from build123d import *

# Parameters (mm, degrees)
ESQUISSE2_R             = 1.2
ENL_V_MAT_EXTRU_1_DEPTH = 16


with BuildPart() as part:
    # Esquisse1 → Révolution1 (revolve)
    with BuildSketch(Plane.XY, mode=Mode.PRIVATE) as r_volution1_sk:
        Polygon((4, 0), (4, -5), (10, -5), (10, -1), (7.75, -1), (7.75, 0), align=None)
    revolve(r_volution1_sk.sketch.rotate(Axis((0, 0, 0), (0, -1, 0)), 180), axis=Axis((0, 0, 0), (0, -1, 0)))

    # Esquisse2 → Enlèv. mat.-Extru.1 (cut, through all)
    with BuildSketch(Plane(origin=(0, 0, 0), x_dir=(1, 0, 0), z_dir=(0, 1, 0))):
        with Locations(Location((6, 0, 0), (0, 0, 180))):
            Circle(ESQUISSE2_R)
        with Locations(Location((-6, 0, 0), (0, 0, 180))):
            Circle(ESQUISSE2_R)
    extrude(amount=-ENL_V_MAT_EXTRU_1_DEPTH, mode=Mode.SUBTRACT)


solid = part.part
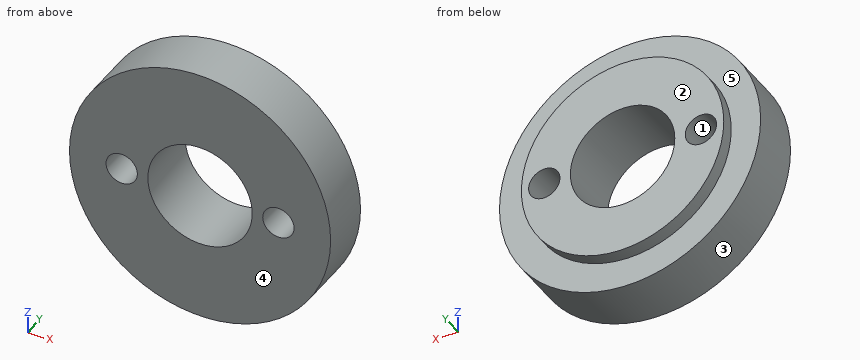
Verification items for the finished model (mm, model axes). Face numbers are marked on the shaded views. A direction names the side the tool comes from. Round coordinates to 2 decimals unless told otherwise and drop trailing zeros. Loops run counter-clockwise (first coordinate to the right, second up) from the corner with the lowest first, then second, coordinate; pieces in that order, holes last. Notation, with made-up numbers: (33, 46) - (68, 46) arc R9 ccw to (68, 61) - close; hole circle Ø6 at (-24, -19.75). An arc over 180 degrees is marked (long way). Use a Markdown table: item, result. Add a question column.
1. Thickness scan on probe 1 along X at (y, z) = (-3.1, 1); probe 2 along Z at (x, y) = (0, -2.75); probe 3 along Y at (x, z) = (-8.25, 3.25). Record the ranges inside material, lowest first. Write a range as [from, to].
2. Section check D-D, the plane y = -2. Record the boundary of the cut face in (x, z).
3. Section check C-C, the plane z = -2. Record the boundary of the cut face in (x, y), plus the area to 3 significant figures.
4. Access from +Z, -Z, +X, -X, +Y, -Y to the whole of each face (thin tool, end or side, straight path). Record for the marked faces 4 and 5.
5. Section check B-B, the plane z = 0. Record the boundary of the cut face in (x, y), plus the area to 3 significant figures.
6. Release check for a two-part mould opening along Z. For the marked faces 1, 2 and 3 record: released by +Z, released by -Z, zero draft, split by the parting line, or undercut.
7. Section check A-A, the plane x = 0. Record the boundary of the cut face in (y, z), plus the area to 3 significant figures.
8. Gauge pin test, flat end, axial feed: pin 1 (3 mm diameter, centred on x = -3, y = -3.5, fed in from +Z). Record the tip position at first contact, or that the pin passes through.
Checks:
| question | item | result |
|---|---|---|
| 1 | probe 1 | x = [-9.95, -6.66], [-5.34, -3.87], [3.87, 5.34], [6.66, 9.95] |
| 1 | probe 2 | z = [-10, -4], [4, 10] |
| 1 | probe 3 | y = [-5, -1] |
| 2 | outline | circle Ø20 at (0, 0); hole circle Ø2.4 at (-6, 0); hole circle Ø8 at (0, 0); hole circle Ø2.4 at (6, 0) |
| 3 | outline | (-9.8, -5) - (-3.46, -5) - (-3.46, 0) - (-7.49, 0) - (-7.49, -1) - (-9.8, -1) - close; (3.46, -5) - (9.8, -5) - (9.8, -1) - (7.49, -1) - (7.49, 0) - (3.46, 0) - close |
| 3 | area | 58.7 mm^2 |
| 4 | face 4 | +Z, -Z, +X, -X, -Y |
| 4 | face 5 | +Y |
| 5 | outline | (-10, -5) - (-7.2, -5) - (-7.2, 0) - (-7.75, 0) - (-7.75, -1) - (-10, -1) - close; (-4.8, -5) - (-4, -5) - (-4, 0) - (-4.8, 0) - close; (4, -5) - (4.8, -5) - (4.8, 0) - (4, 0) - close; (7.2, -5) - (10, -5) - (10, -1) - (7.75, -1) - (7.75, 0) - (7.2, 0) - close |
| 5 | area | 31.5 mm^2 |
| 6 | face 1 | undercut |
| 6 | face 2 | zero draft |
| 6 | face 3 | split by the parting line |
| 7 | outline | (-5, -10) - (-1, -10) - (-1, -7.75) - (0, -7.75) - (0, -4) - (-5, -4) - close; (-5, 4) - (0, 4) - (0, 7.75) - (-1, 7.75) - (-1, 10) - (-5, 10) - close |
| 7 | area | 55.5 mm^2 |
| 8 | pin 1 | stops at z = 9.89 |
